Could you check a few things on this model? Use its own coordinates, in mm. Face numbers are marked on the shaded views. A direction names the side the tool comes from. Round coordinates to 2 decimals unless told otherwise and drop trailing zeros. Loops run counter-clockwise (first coordinate to the right, second up) from the corner with the lowest first, then second, coordinate; pieces in that order, holes last. Notation, with made-up numbers: M 31,-32.75 L 87,-32.75 A27 cw 87,-12.75 Z; hole C 26,47 d10. An arc over 180 degrees is marked long. Answer in a Markdown table with one row per item.
```python
from build123d import *

# Parameters (mm, degrees)
F1_DEPTH = 2.54


with BuildPart() as f1:
    # F0 (on Front) → F1 (new body)
    with BuildSketch(Plane.XZ):
        with BuildLine():
            Line((6.083285, -1.316122), (6.083285, 1.316122))
            Line((6.083285, 1.316122), (3.594506, 1.316122))
            ThreePointArc((3.594506, 1.316122), (3.295386, -0.119464), (2.447808, -1.316122))
            Line((2.447808, -1.316122), (6.083285, -1.316122))
        make_face()
        with BuildLine():
            ThreePointArc((2.447808, -1.316122), (3.295386, -0.119464), (3.594506, 1.316122))
            Line((3.594506, 1.316122), (2.0701, 1.316122))
            ThreePointArc((2.0701, 1.316122), (0, -0.753978), (-2.0701, 1.316122))
            Line((-2.0701, 1.316122), (-3.594506, 1.316122))
            ThreePointArc((-3.594506, 1.316122), (-3.295386, -0.119464), (-2.447808, -1.316122))
            Line((-2.447808, -1.316122), (2.447808, -1.316122))
        make_face()
        with BuildLine():
            Line((2.0701, 1.316122), (3.594506, 1.316122))
            ThreePointArc((3.594506, 1.316122), (0, 4.910627), (-3.594506, 1.316122))
            Line((-3.594506, 1.316122), (-2.0701, 1.316122))
            ThreePointArc((-2.0701, 1.316122), (0, 3.386222), (2.0701, 1.316122))
        make_face()
        with BuildLine():
            ThreePointArc((-2.447808, -1.316122), (-3.295386, -0.119464), (-3.594506, 1.316122))
            Line((-3.594506, 1.316122), (-6.083285, 1.316122))
            Line((-6.083285, 1.316122), (-6.083285, -1.316122))
            Line((-6.083285, -1.316122), (-2.447808, -1.316122))
        make_face()
    extrude(amount=F1_DEPTH)


solid = f1.part
```
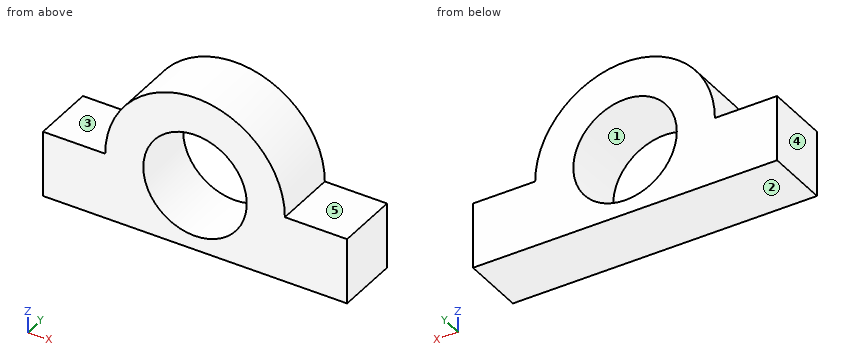
1) Will these pins go through, and if not, where does the flat tip stop? P1, Ø1, axis at x = 4.5, y = -0.5, coming from the +Z side; P2, Ø1, axis at x = -2, y = -0.5, coming from the +Z side.
Computed:
| item | result |
|---|---|
| P1 | stops at z = 1.32 |
| P2 | stops at z = 4.58 |
2) I want a section at B-B, the plane y = -1.2. Please give me the cut outline in (x, z).
Computed:
| item | result |
|---|---|
| outline | M -6.08,-1.32 L 6.08,-1.32 L 6.08,1.32 L 3.59,1.32 A3.59 ccw -3.59,1.32 L -6.08,1.32 Z; hole C 0,1.32 d4.14 |
3) I need wall thicknesses on line 1 (Z direction, x = 0, y = -1); line 2 (Z direction, x = 4, y = -1.8); line 3 (X direction, y = -0.85, z = 2.25). Which ranges of each line are inside material? Lowest first, please.
Computed:
| item | result |
|---|---|
| line 1 | z = -1.32 to -0.75, 3.39 to 4.91 |
| line 2 | z = -1.32 to 1.32 |
| line 3 | x = -3.47 to -1.85, 1.85 to 3.47 |
4) I want a section at A-A, the plane x = 0. Please give me the cut outline in (y, z), plus the area to 3 significant figures.
Computed:
| item | result |
|---|---|
| outline | M -2.54,-1.32 L 0,-1.32 L 0,-0.75 L -2.54,-0.75 Z; M -2.54,3.39 L 0,3.39 L 0,4.91 L -2.54,4.91 Z |
| area | 5.30 mm² |
5) Which directions (+Z, -Z, +X, -X, +Y, -Y) give clear straight access to the entire face, cutting with the end or side of a thin tool? Please do the marked faces 4 and 5.
Computed:
| item | result |
|---|---|
| face 4 | +Z, -Z, -X, +Y, -Y |
| face 5 | +Z, +X, +Y, -Y |
6) If we mould it in two halves opening along Z, with no side actions, what happens to the marked faces 1, 2 and 3? For each: released by +Z, released by -Z, zero draft, split by the parting line, or undercut.
Computed:
| item | result |
|---|---|
| face 1 | undercut |
| face 2 | released by -Z |
| face 3 | released by +Z |
7) I want a section at C-C, the plane z = 0. Please give me the cut outline in (x, y).
Computed:
| item | result |
|---|---|
| outline | M -6.08,-2.54 L -1.6,-2.54 L -1.6,0 L -6.08,0 Z; M 1.6,-2.54 L 6.08,-2.54 L 6.08,0 L 1.6,0 Z |
8) I want a section at D-D, the plane x = -4.5. Please give me the cut outline in (y, z), plus the area to 3 significant figures.
Computed:
| item | result |
|---|---|
| outline | M -2.54,-1.32 L 0,-1.32 L 0,1.32 L -2.54,1.32 Z |
| area | 6.69 mm² |
